Geometry: final body of the model. Coordinates: model frame, mm. A direction names the side the tool comes from. Round coordinates to 2 decimals unless told otherwise and drop trailing zeros. Write each loop counter-clockwise with the first axis right and the second up, starting at its lowest first coordinate (ties: lowest second). Pieces come first, ordered by that corner, then holes. Notation, with made-up numbers: (68, 5.5) - (83, 5.5) arc R23 cw to (83, 40.5) - close; hole circle Ø11 at (-31, -24.5). An arc over 180 degrees is marked (long way). Use a Markdown table: item, result. Add a question column.
```python
from build123d import *


with BuildPart() as part:
    # Эскиз1 → Повернуть1 (revolve)
    with BuildSketch(Plane(origin=(0, 0, 0), x_dir=(0, 0, -1), z_dir=(1, 0, 0))):
        Polygon((1.5, 2), (-1.5, 2), (-1.5, 2.657142857), (-1.2, 2.657142857), (-1.2, 3.342857143), (-1.5, 3.342857143), (-1.5, 4), (1.5, 4), (1.5, 3.342857143), (1.2, 3.342857143), (1.2, 2.657142857), (1.5, 2.657142857), align=None)
        with BuildLine():
            Line((0.492391084, 3.342857143), (1, 3.342857143))
            Line((1, 3.342857143), (1, 2.657142857))
            Line((1, 2.657142857), (0.492391084, 2.657142857))
            ThreePointArc((0.492391084, 2.657142857), (0, 2.4), (-0.492391084, 2.657142857))
            Line((-0.492391084, 2.657142857), (-1, 2.657142857))
            Line((-1, 2.657142857), (-1, 3.342857143))
            Line((-1, 3.342857143), (-0.492391084, 3.342857143))
            ThreePointArc((-0.492391084, 3.342857143), (0, 3.6), (0.492391084, 3.342857143))
        make_face(mode=Mode.SUBTRACT)
    revolve(axis=Axis((0, 0, 0), (0, 0, -1)))


solid = part.part
```
1) Section A-A, the plane x = 0. State how many separate pieces and enclosed holes the cut face has, then the cut area to 3 significant figures.
2) Set-up query: faces 1 (the flat face through (-3, 0, 1.2)), 2 (the flat face through (-3, 0, -1.2)), 3 (the flat face through (-3, 0, -1)). Return all of +Z, -Z, +X, -X, +Y, -Y with unobstructed straight access to the full face (end or side cutting, diameter ignored); none if empty.
3) Section C-C, the plane z = 0.2. Return the cut outline in (x, y).
4) Section D-D, the plane z = -0.3. Return the cut outline in (x, y), then the cut area to 3 significant figures.
5) Material intervals for L1, parallel to X at y = 0, z = -0.7; L2, parallel to Y at x = 2.25, z = 0.9; L3, parallel to Y at x = 1, z = 0.8, sorted ascending. Write a range as from..to.
6) Draft query along Z for faces 4 (the cylindrical face through (1.796, -1.958, -0.743)), 5 (the flat face through (-3, 2, -1.5)), 6 (the flat face through (2, -1, 1.5)). Return one class per face: released by +Z, released by -Z, zero draft, split by the parting line, or undercut.
7) Pin query (flat end, axial travel): P1, Ø3, axis at x = 0, y = 0, coming from the -Z side; P2, Ø1.5, axis at y = 1, z = -1, coming from the +X side; P3, Ø1, axis at y = 1.5, z = 1, coming from the -X side. Return the tip coordinate at first contact, or that it passes through.
Output values:
| question | item | result |
|---|---|---|
| 1 | separate pieces | 2 |
| 1 | enclosed holes | 2 |
| 1 | area | 7.72 mm^2 |
| 2 | face 1 | +Z |
| 2 | face 2 | -Z |
| 2 | face 3 | none |
| 3 | outline | circle Ø8 at (0, 0); circle Ø4.87 at (0, 0); hole circle Ø7.13 at (0, 0); hole circle Ø4 at (0, 0) |
| 4 | outline | circle Ø8 at (0, 0); circle Ø4.96 at (0, 0); hole circle Ø7.04 at (0, 0); hole circle Ø4 at (0, 0) |
| 4 | area | 18.1 mm^2 |
| 5 | L1 | x = -4..-3.34, -2.66..-2, 2..2.66, 3.34..4 |
| 5 | L2 | y = -3.31..-2.47, -1.41..1.41, 2.47..3.31 |
| 5 | L3 | y = -3.87..-3.19, -2.46..-1.73, 1.73..2.46, 3.19..3.87 |
| 6 | face 4 | undercut |
| 6 | face 5 | released by -Z |
| 6 | face 6 | released by +Z |
| 7 | P1 | passes through |
| 7 | P2 | stops at x = 3.99 |
| 7 | P3 | stops at x = -3.87 |
